Build history of the part. All positions in model axes, mm. Face numbers are marked on the shaded views. A direction names the side the tool comes from. Round coordinates to 2 decimals unless told otherwise and drop trailing zeros. Write each loop counter-clockwise with the first axis right and the second up, starting at its lowest first coordinate (ties: lowest second). Pieces come first, ordered by that corner, then holes. Notation, with made-up numbers: M -2,12.25 L 35,12.25 A31 ccw 35,45.25 Z; hole C 35,-39.5 d6. An arc over 180 degrees is marked long. Write item = value, one per line.
from build123d import *

# Parameters (mm, degrees)
EXTRUDE_1_DEPTH     = 10
CUT_EXTRUDE_1_REACH = 21.9
SKETCH_3_R          = 3
SKETCH_4_W          = 10
SKETCH_4_H          = 8
EXTRUDE_2_DEPTH     = 16


with BuildPart() as part:
    # 草图2 → 凸台-拉伸1 (new body)
    with BuildSketch(Plane(origin=(0, 0, 95), x_dir=(-1, 0, 0), z_dir=(0, 0, -1))):
        Polygon((2, -10), (12, -10), (12, -8), (14, -8), (14, 0), (0, 0), (0, -8), (2, -8), align=None)
    extrude(amount=EXTRUDE_1_DEPTH)

    # 草图3 → 切除-拉伸1 (cut, up to next)
    with BuildSketch(Plane(origin=(0, 0, 85), x_dir=(-1, 0, 0), z_dir=(0, 0, -1)), mode=Mode.PRIVATE) as cut_extrude_1_sk1:
        with Locations((7, -5)):
            Circle(SKETCH_3_R)
    cut_extrude_1_tool1 = extrude(cut_extrude_1_sk1.sketch, amount=-CUT_EXTRUDE_1_REACH, mode=Mode.PRIVATE) & part.part
    add(cut_extrude_1_tool1.solids().sort_by_distance((-7, -5, 85))[0], mode=Mode.SUBTRACT)

    # 草图4 → 凸台-拉伸2 (add)
    with BuildSketch(Plane(origin=(0, 0, 0), x_dir=(0, 0, -1), z_dir=(1, 0, 0))):
        with Locations((-90, -4)):
            Rectangle(SKETCH_4_W, SKETCH_4_H)
    extrude(amount=EXTRUDE_2_DEPTH)


solid = part.part
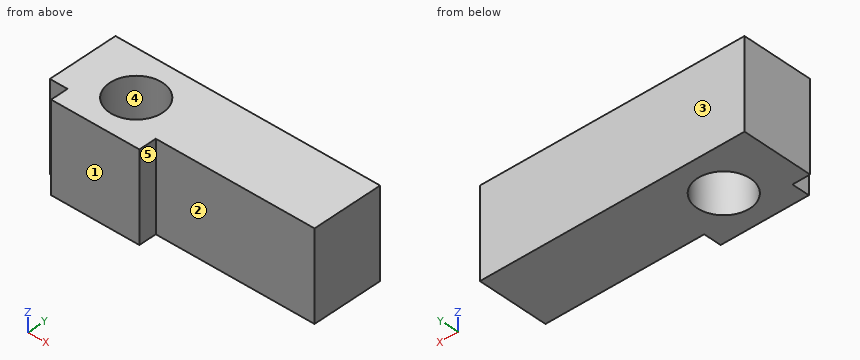
1. Tool access for the marked faces 1 and 2: list every direction of +Z, -Z, +X, -X, +Y, -Y with a clear straight run to the whole face (end or side of a thin tool).
Responses:
face_1 = +Z, -Z, +X, -X, -Y
face_2 = +Z, -Z, +X, -Y
2. Band-saw the part on D-D (x = -0.75). List the corners of the cut face in (y, z).
Responses:
outline = M -8,85 L 0,85 L 0,95 L -8,95 Z
3. Band-saw the part on C-C (z = 93.5). List the corners of the cut face in (x, y).
Responses:
outline = M -14,-8 L -12,-8 L -12,-10 L -2,-10 L -2,-8 L 16,-8 L 16,0 L -14,0 Z; hole C -7,-5 d6
4. Flat gauge pins, fed straight in: pin 1 (2 mm diameter, centred on x = 5.5, z = 90.5, fed in from -Y); pin 2 (1.6 mm diameter, centred on y = -9, z = 92, fed in from +X); pin 3 (0.6 mm diameter, centred on y = -9.5, z = 92.5, fed in from -X). Where does each tip first touch, or does it go through?
Responses:
pin_1 = -8
pin_2 = -2
pin_3 = -12
5. Band-saw the part on A-A (x = -7). List the corners of the cut face in (y, z), plus the area to 3 significant figures.
Responses:
outline = M -10,85 L -8,85 L -8,95 L -10,95 Z; M -2,85 L 0,85 L 0,95 L -2,95 Z
area = 40.0 mm²
6. Probe probe 1 along Y at (x, z) = (-7, 91.5); probe 2 along Y at (x, z) = (4, 93); probe 3 along X at (y, z) = (-6.75, 92.75). List the from-to ranges inside material, lowest first.
Responses:
probe_1 = -10 to -8, -2 to 0
probe_2 = -8 to 0
probe_3 = -14 to -9.44, -4.56 to 16
7. Band-saw the part on B-B (y = -5). List the corners of the cut face in (x, z).
Responses:
outline = M -14,85 L -10,85 L -10,95 L -14,95 Z; M -4,85 L 16,85 L 16,95 L -4,95 Z
8. Mould opens along X. For the marked faces 3, 4 and 5 say: pulls with the +X half, pulls with the -X half, needs draft (parallel to the pull), parting line crosses it, or undercut.
Responses:
face_3 = needs draft
face_4 = undercut
face_5 = pulls with the +X half
